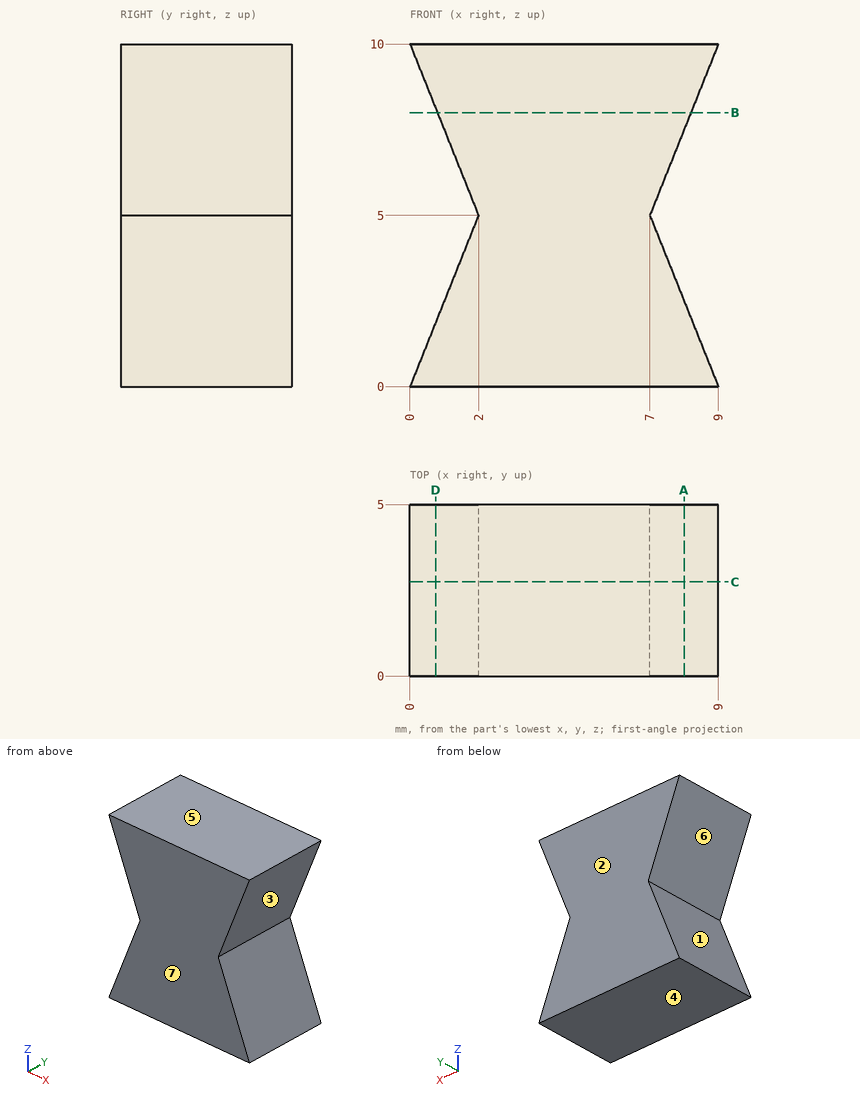
Geometry: see drawing. Coordinates: mm, zero at the bounding-box minimum. A direction names the side the tool comes from. Give positions to 0.01 mm unless a question says otherwise; leave off trailing zeros. Loops run counter-clockwise (first coordinate to the right, second up) from the corner with the lowest first, then second, coordinate; pieces in that order, holes last. Notation, with made-up numbers: M 75,16 L 119,16 A32 cw 119,50 Z; hole C 89.25,7 d4. An arc over 180 degrees is marked long. Answer as CSV lines item,"result". Start each with the question number.
1. Section A-A on x = 8. Return loops of the section in (y, z).
2. Pull-direction query (Z, two-part tool) for the marked faces 4, 5, 6 and 7; classes: released by +Z, released by -Z, zero draft, split by the parting line, or undercut.
3. Section D-D on x = 0.75. Return loops of the section in (y, z) (3 decimals).
4. Line query: L1, parallel to Z at x = 8.5, y = 1.95; L2, parallel to X at y = 1.55, z = 3.5; L3, parallel to X at y = 4.3, z = 3.25. Output: solid intervals per line, ascending.
5. Reachability of the marked faces 1, 2 and 3 from +Z, -Z, +X, -X, +Y, -Y: full face, straight path, thin tool, end or side. Return the list, or none.
6. Section C-C on y = 2.75. Return loops of the section in (x, z), plus the area to 3 significant figures.
7. Section B-B on z = 8. Return loops of the section in (x, y), plus the area to 3 significant figures.
Computed values:
1,outline,"M 0,0 L 5,0 L 5,2.5 L 0,2.5 Z; M 0,7.5 L 5,7.5 L 5,10 L 0,10 Z"
2,face 4,"released by -Z"
2,face 5,"released by +Z"
2,face 6,"undercut"
2,face 7,"zero draft"
3,outline,"M 0,0 L 5,0 L 5,1.875 L 0,1.875 Z; M 0,8.125 L 5,8.125 L 5,10 L 0,10 Z"
4,L1,"z = 0 to 1.25, 8.75 to 10"
4,L2,"x = 1.4 to 7.6"
4,L3,"x = 1.3 to 7.7"
5,face 1,"-X, +Y, -Y"
5,face 2,"+Z, -Z, +X, -X, +Y"
5,face 3,"+X, +Y, -Y"
6,outline,"M 0,0 L 9,0 L 7,5 L 9,10 L 0,10 L 2,5 Z"
6,area,"70.0 mm²"
7,outline,"M 0.8,0 L 8.2,0 L 8.2,5 L 0.8,5 Z"
7,area,"37.0 mm²"
